Verification items for the finished model (mm, model axes). A direction names the side the tool comes from. Round coordinates to 2 decimals unless told otherwise and drop trailing zeros. Order: outer loops, then holes, each group sorted by start corner. A loop starts at its lowest first (then second) coordinate and runs counter-clockwise, first axis right, second up. Notation, with made-up numbers: (-9, 46.5) -> (24, 46.5) arc R28 ccw to (24, 72.5) -> close; hole circle Ø3 at (67.25, 66.5). An arc over 180 degrees is marked (long way). Return JSON: item names as keys, results as strings. Group by question number.
Item 1: Sectioned sample at B-B on z = 21.25. Record the cut outline in (x, y), plus the area to 3 significant figures.
Item 2: Scan lines: probe 1 along Z at (x, y) = (-2, 2.5); probe 2 along X at (y, z) = (0, 21.5); probe 3 along Z at (x, y) = (4, 3.5). Record each from-to range of solid material in increasing order. Write a range as from..to.
Item 3: Draft check along Z on faces 4 (the flat face through (0, -4, 7.62)), 5 (the flat face through (0.126, -5.048, 3.757)), 6 (the flat face through (0, 0, 23.812)). Enter one of: pulls with the +Z half, pulls with the -Z half, needs draft (parallel to the pull), parting line crosses it, or undercut.
Item 4: Depth check by flat-ended pin: pin 1 Ø1.6 at (x, y) = (0, 4.5) entering from -Z; pin 2 Ø4 at (x, z) = (3, 12) entering from -Y; pin 3 Ø2 at (x, z) = (0.5, 13.5) entering from -Y; pin 4 Ø1.5 at (y, z) = (-3, 22.5) entering from +X. Enter the tip coordinate at first touch or a pass-through.
Item 5: Sectioned sample at C-C on x = 1.5. Record the cut outline in (y, z).
Item 6: Sectioned sample at D-D on x = 2.75. Record the cut outline in (y, z), plus the area to 3 significant figures.
Item 7: Sectioned sample at A-A on y = 0. Record the cut outline in (x, z), plus the area to 3 significant figures.
Item 8: Access from +Z, -Z, +X, -X, +Y, -Y to the whole of each face (thin tool, end or side, straight path). Record for faces 1 (the cylindrical face through (-4.063, 0.089, 22.247)), 2 (the flat face through (-5.334, 0, 13)), 3 (the flat face through (0, 4, 7.62)).
```python
from build123d import *

# Parameters (mm, degrees)
F1_DEPTH = 25.4
F2_R     = 4.064
F3_DEPTH = 4.7625
F4_W     = 8.128
F4_H     = 3.302
F5_DEPTH = 5.335
F6_R     = 4.064
F7_DEPTH = 1.5875
F9_DEPTH = 7.62


with BuildPart() as f1:
    # F0 (on Top) → F1 (new body)
    with BuildSketch(Plane.XY):
        Polygon((5.334, -3.079586), (5.334, 3.079586), (0, 6.159173), (-5.334, 3.079586), (-5.334, -3.079586), (0, -6.159173), align=None)
    extrude(amount=F1_DEPTH)

    # F2 (on face) → F3 (cut)
    with BuildSketch(Plane.XY.offset(25.4)):
        Circle(F2_R)
    extrude(amount=-F3_DEPTH, mode=Mode.SUBTRACT)

    # F4 (on Right) → F5 (cut, through all)
    with BuildSketch(Plane.YZ):
        with Locations((0, 22.2885)):
            Rectangle(F4_W, F4_H)
    extrude(amount=F5_DEPTH, mode=Mode.SUBTRACT)

    # F6 (on face) → F7 (join)
    with BuildSketch(Plane.XY.offset(25.4)):
        Circle(F6_R)
    extrude(amount=-F7_DEPTH)

    # F8 (on face) → F9 (cut)
    with BuildSketch(Plane(origin=(0, 0, 0), x_dir=(1, 0, 0), z_dir=(0, 0, -1))):
        Polygon((0.559566, -4.962233), (0.664833, -4.072655), (-0.148677, -3.697645), (-0.75672, -4.355455), (-0.319002, -5.137013), align=None)
        Polygon((-0.148677, 3.697645), (0.664833, 4.072655), (0.559566, 4.962233), (-0.319002, 5.137013), (-0.75672, 4.355455), align=None)
    extrude(amount=-F9_DEPTH, mode=Mode.SUBTRACT)


solid = f1.part
```
Recorded:
{
 "1": {"outline": "(-5.33, -3.08) -> (0, -6.16) -> (3.63, -4.06) -> (0, -4.06) arc R4.06 cw to (0, 4.06) -> (3.63, 4.06) -> (0, 6.16) -> (-5.33, 3.08) -> close", "area": "30.9 mm²"},
 "2": {"probe 1": "0..20.64, 23.81..25.4", "probe 2": "-5.33..-4.06", "probe 3": "0..20.64, 23.94..25.4"},
 "3": {"face 4": "pulls with the -Z half", "face 5": "needs draft", "face 6": "undercut"},
 "4": {"pin 1": "z = 0", "pin 2": "y = -5.58", "pin 3": "y = -6.16", "pin 4": "x = -1.57"},
 "5": {"outline": "(-5.29, 0) -> (5.29, 0) -> (5.29, 25.4) -> (-5.29, 25.4) -> close; hole (-4.06, 20.64) -> (4.06, 20.64) -> (4.06, 23.94) -> (3.78, 23.94) -> (3.78, 23.81) -> (-3.78, 23.81) -> (-3.78, 23.94) -> (-4.06, 23.94) -> close"},
 "6": {"outline": "(-4.57, 0) -> (4.57, 0) -> (4.57, 25.4) -> (-4.57, 25.4) -> close; hole (-4.06, 20.64) -> (4.06, 20.64) -> (4.06, 23.94) -> (2.99, 23.94) -> (2.99, 23.81) -> (-2.99, 23.81) -> (-2.99, 23.94) -> (-4.06, 23.94) -> close", "area": "206 mm²"},
 "7": {"outline": "(-5.33, 0) -> (5.33, 0) -> (5.33, 20.64) -> (-4.06, 20.64) -> (-4.06, 23.81) -> (4.06, 23.81) -> (4.06, 23.94) -> (5.33, 23.94) -> (5.33, 25.4) -> (-5.33, 25.4) -> close", "area": "241 mm²"},
 "8": {"face 1": "+X", "face 2": "+Z, -Z, -X, +Y, -Y", "face 3": "-Z"}
}
